from build123d import *

# Parameters (mm, degrees)
F0_R     = 11
F1_DEPTH = 17
F2_R     = 2.5
F3_DEPTH = 6.001


with BuildPart() as f1:
    # F0 (on Front) → F1 (new body)
    with BuildSketch(Plane.XZ):
        with BuildLine():
            ThreePointArc((-15, 0), (0, -15), (15, 0))
            ThreePointArc((15, 0), (0, 15), (-15, 0))
        make_face()
        Circle(F0_R, mode=Mode.SUBTRACT)
        with BuildLine():
            Line((15, -11), (15, 0))
            ThreePointArc((15, 0), (0, -15), (-15, 0))
            Line((-15, 0), (-15, -11))
            Line((-15, -11), (-25, -11))
            Line((-25, -11), (-25, -17))
            Line((-25, -17), (25, -17))
            Line((25, -17), (25, -11))
            Line((25, -11), (15, -11))
        make_face()
    extrude(amount=F1_DEPTH)

    # F2 (on face) → F3 (cut, through all)
    with BuildSketch(Plane.XY.offset(-11)):
        with Locations((-20, -8.5)):
            Circle(F2_R)
        with Locations((20, -8.5)):
            Circle(F2_R)
    extrude(amount=-F3_DEPTH, mode=Mode.SUBTRACT)


solid = f1.part
Verification items for the finished model (mm, model axes). A direction names the side the tool comes from. Coordinates: 2 decimals unless noted, no trailing zeros. Loops run counter-clockwise (first coordinate to the right, second up) from the corner with the lowest first, then second, coordinate; pieces in that order, holes last. Notation, with made-up numbers: (67.5, 73) -> (119.5, 73) arc R20 ccw to (119.5, 89) -> close; hole circle Ø2 at (-22.75, 48.25). An arc over 180 degrees is marked (long way). Answer as a JSON object with one key per item and string values. Group by question number.
Item 1: Tool access check on faces 5 (the flat face through (-18, -6, -11)), 6 (the flat face through (15, -8, -6)), 7 (the cylindrical face through (-22, -10, -14)). Record the directions out of +Z, -Z, +X, -X, +Y, -Y that give a thin tool (end or side, any length) a straight path to the whole face; none if there is none.
Item 2: Sectioned sample at B-B on z = 10.5. Record the boundary of the cut face in (x, y), plus the area to 3 significant figures.
Item 3: Sectioned sample at C-C on y = -5.5. Record the boundary of the cut face in (x, z).
Item 4: Mould release check, pull along Y, two halves, no side actions. Record for faces 1 (the flat face through (-0.4, 0, -11.4)), 2 (the flat face through (25, -8, -14)), 3 (the flat face through (-0.4, -17, -11.4)), 4 (the cylindrical face through (18, -10, -14)): +Y half, -Y half, draft (parallel to the pull), parting line (faces both ways), or undercut.
Item 5: Sectioned sample at D-D on x = 13.5. Record the boundary of the cut face in (y, z), plus the area to 3 significant figures.
Item 6: Scan lines: probe 1 along X at (y, z) = (-10.5, 10); probe 2 along X at (y, z) = (-9.75, 7); probe 3 along Z at (x, y) = (-3, -11.25). Record each from-to range of solid material in increasing order.
Item 7: Depth check by flat-ended pin: pin 1 (9 mm diameter, centred on y = -12, z = -6, fed in from -X); pin 2 (5.5 mm diameter, centred on y = -10, z = -8, fed in from +X); pin 3 (5 mm diameter, centred on x = -19.5, y = -10.5, fed in from +Z); pin 4 (3 mm diameter, centred on x = 20, y = -8.5, fed in from -Z). Enter the tip coordinate at first touch or a pass-through.
Item 8: Sectioned sample at A-A on x = -20. Record the boundary of the cut face in (y, z), plus the area to 3 significant figures.
Evaluation:
{
 "1": {"face 5": "+Z, -X, +Y, -Y", "face 6": "+Z, +X, +Y, -Y", "face 7": "+Z, -Z"},
 "2": {"outline": "(-10.71, -17) -> (-3.28, -17) -> (-3.28, 0) -> (-10.71, 0) -> close; (3.28, -17) -> (10.71, -17) -> (10.71, 0) -> (3.28, 0) -> close", "area": "253 mm²"},
 "3": {"outline": "(-25, -17) -> (25, -17) -> (25, -11) -> (15, -11) -> (15, 0) arc R15 ccw to (-15, 0) -> (-15, -11) -> (-25, -11) -> close; hole circle Ø22 at (0, 0)"},
 "4": {"face 1": "+Y half", "face 2": "draft", "face 3": "-Y half", "face 4": "undercut"},
 "5": {"outline": "(-17, -17) -> (0, -17) -> (0, 6.54) -> (-17, 6.54) -> close", "area": "400 mm²"},
 "6": {"probe 1": "x = -11.18 to -4.58, 4.58 to 11.18", "probe 2": "x = -13.27 to -8.49, 8.49 to 13.27", "probe 3": "z = -17 to -10.58, 10.58 to 14.7"},
 "7": {"pin 1": "stops at x = -15", "pin 2": "stops at x = 15", "pin 3": "stops at z = -11", "pin 4": "passes through"},
 "8": {"outline": "(-17, -17) -> (-11, -17) -> (-11, -11) -> (-17, -11) -> close; (-6, -17) -> (0, -17) -> (0, -11) -> (-6, -11) -> close", "area": "72.0 mm²"}
}
